Solid Edge part; units mm, degrees
sketch "Sketch1" plane through (0, 0, 0) normal (1, 0, 0) x (0, 1, 0)
  line L0 (0, 0) -> (7, 0)
  line L1 (7, 0) -> (7, 30)
  arc A0 (7, 30) -> (13.2834, 36.9632) centre (14, 30) cw
  line L2 (32.7166, 38.9632) -> (13.2834, 36.9632)
  arc A1 (39, 45.9264) -> (32.7166, 38.9632) centre (32, 45.9264) cw
  line L3 (39, 45.9264) -> (39, 71.9264)
  line L4 (39, 71.9264) -> (32, 71.9264)
  line L5 (32, 71.9264) -> (32, 54.9264)
  arc A2 (25, 47.9264) -> (32, 54.9264) centre (25, 54.9264) ccw
  line L6 (25, 47.9264) -> (7, 47.9264)
  arc A3 (7, 47.9264) -> (0, 40.9264) centre (7, 40.9264) ccw
  line L7 (0, 40.9264) -> (0, 0)
  dimension "D1" = 39
  dimension "D2" = 7
  dimension "D3" = 32.7166
extrude "Protrusion1" add sketch "Sketch1" along normal mid plane 120
sketch "Sketch2" plane through (0, 0, 25.1762) normal (0, -1, 0) x (1, 0, 0)
  circle A0 centre (0, -4.1762) radius 1.7
  circle A1 centre (0, -20.1762) radius 1.7
  circle A2 centre (-50, 34.7502) radius 1.7
  circle A3 centre (50, 34.7502) radius 1.7
extrude "Cutout1" cut sketch "Sketch2" against normal through all
sketch "Sketch3" plane through (0, 0, 0) normal (0, -1, 0) x (1, 0, 0)
  line L0 (-14, 0) -> (-14, 23.2382)
  arc A0 (-19.1896, 30) -> (-14, 23.2382) centre (-21, 23.2382) cw
  line L1 (-19.1896, 30) -> (-60, 40.9264)
  line L2 (-60, 40.9264) -> (-101.8817, 40.9264)
  line L3 (-101.8817, 40.9264) -> (-101.8817, -44.3186)
  line L4 (-101.8817, -44.3186) -> (159.9543, -44.3186)
  line L5 (159.9543, -44.3186) -> (159.9543, 40.9264)
  line L6 (159.9543, 40.9264) -> (60, 40.9264)
  line L7 (60, 40.9264) -> (19.1896, 30)
  arc A1 (14, 23.2382) -> (19.1896, 30) centre (21, 23.2382) cw
  line L8 (14, 23.2382) -> (14, 0)
  line L9 (14, 0) -> (-14, 0)
  dimension "D1" = 14
  dimension "D2" = 19.1896
extrude "Cutout2" cut sketch "Sketch3" against normal through all
The model under review builds one solid part; all positions refer to its coordinate system, in mm. A direction names the side the tool comes from. Give positions to 0.01 mm unless a question says otherwise; leave off trailing zeros. Write each loop counter-clockwise with the first axis right and the second up, starting at its lowest first coordinate (ties: lowest second). Pieces come first, ordered by that corner, then holes.
1. Add section A-A, the plane z = 5. Write out the cut boundary in (x, y), plus the area to 3 significant figures.
2. For P1, Ø8, axis at x = -31, y = 13.5, coming from the -Z side; P2, Ø2, axis at x = -48, y = 27.5, coming from the +Z side; P3, Ø24, axis at x = -9.5, z = 10.5, coming from the +Y side, all flat-tipped, find the tip position at first contact; note any pin that passes through.
3. Draft analysis for pull direction Z (two halves, no side actions). For faces 1 (the flat face through (-1, 16, 47.926)), 2 (the cylindrical face through (-0.221, 3.451, 22.686)), 3 (the flat face through (0, 0, 25)), state which applies: +Z half, -Z half, draft (parallel to the pull), parting line (faces both ways), or undercut.
4. Add section D-D, the plane x = -50. Write out the cut boundary in (y, z), plus the area to 3 significant figures.
5. Add section B-B, the plane x = 0. Write out the cut boundary in (y, z), plus the area to 3 significant figures.
6. Tool access review of faces 4 (the flat face through (60, 28, 46)), 5 (the flat face through (-14, 3, 11)): name each direction out of +Z, -Z, +X, -X, +Y, -Y from which nothing blocks a thin tool from reaching the whole face with its end or side.
7. Add section C-C, the plane x = 41. Write out the cut boundary in (y, z), plus the area to 3 significant figures.
8. Wall thickness on L1, parallel to Z at x = 0, y = 3; L2, parallel to Z at x = 0, y = 2; L3, parallel to X at y = 6, z = 4.5: over which ranges is each line inside the solid? List them lowest first.
Worked answers:
1. outline: (-14, 0) - (-1.7, 0) - (-1.7, 7) - (-14, 7) - close; (1.7, 0) - (14, 0) - (14, 7) - (1.7, 7) - close
1. area: 172 mm2
2. P1: stops at z = 35.36
2. P2: stops at z = 48.86
2. P3: stops at y = 7
3. face 1: +Z half
3. face 2: undercut
3. face 3: draft
4. outline: (0, 38.25) - (25.78, 38.25) - (32.72, 38.96) arc R7 ccw to (39, 45.93) - (39, 58.23) - (32, 58.23) - (32, 54.93) arc R7 cw to (25, 47.93) - (7, 47.93) arc R7 ccw to (0, 40.93) - close; (32, 61.63) - (39, 61.63) - (39, 71.93) - (32, 71.93) - close
4. area: 504 mm2
5. outline: (0, 0) - (7, 0) - (7, 3.3) - (0, 3.3) - close; (0, 6.7) - (7, 6.7) - (7, 19.3) - (0, 19.3) - close; (0, 22.7) - (7, 22.7) - (7, 30) arc R7 cw to (13.28, 36.96) - (32.72, 38.96) arc R7 ccw to (39, 45.93) - (39, 71.93) - (32, 71.93) - (32, 54.93) arc R7 cw to (25, 47.93) - (7, 47.93) arc R7 ccw to (0, 40.93) - close
5. area: 775 mm2
6. face 4: +Z, -Z, +X, +Y, -Y
6. face 5: -Z, -X, +Y, -Y
7. outline: (0, 35.84) - (10.14, 35.84) arc R7 cw to (13.28, 36.96) - (32.72, 38.96) arc R7 ccw to (39, 45.93) - (39, 71.93) - (32, 71.93) - (32, 54.93) arc R7 cw to (25, 47.93) - (7, 47.93) arc R7 ccw to (0, 40.93) - close
7. area: 566 mm2
8. L1: z = 0 to 3.3, 6.7 to 19.3, 22.7 to 46.67
8. L2: z = 0 to 3.3, 6.7 to 19.3, 22.7 to 45.83
8. L3: x = -14 to -1.62, 1.62 to 14
